For this review, take the finished solid that the model builds, in its own axes (mm). A direction names the side the tool comes from. Give positions to 0.01 mm unless a question says otherwise; leave off trailing zeros. Write each loop counter-clockwise with the first axis right and the second up, starting at its lowest first coordinate (ties: lowest second). Pieces come first, ordered by that corner, then holes.
Q1. We need section D-D (z = 0.1). Write out the cut boundary in (x, y).
Q2. We need section C-C (x = 1.1). Write out the cut boundary in (y, z).
Q3. We need section A-A (z = -3.55). Write out the cut boundary in (x, y) (3 decimals).
Q4. For line 1 (Y direction, x = -0.5, z = -4.15); line 2 (Y direction, x = -0.3, z = -2.25); line 3 (Z direction, x = 0, y = 1), list the stretches that pass through material, from the lowest coordinate up.
Q5. Machinability: for faces 5 (the flat face through (0.5, 7.3, -2.75)), 6 (the flat face through (0, 3, -0.75)), 7 (the flat face through (-0.5, 3, 0)), which of the approach directions +Z, -Z, +X, -X, +Y, -Y give a long, thin tool a straight path to every point of the face, cutting with its end or side? Answer none if there is none.
Q6. Mouldability with a two-part tool opening along Z and no side actions: class faces 1 (the cylindrical face through (-0.133, 1.479, -0.167)), 2 (the flat face through (0.5, 3, 0)), 3 (the flat face through (-1.25, 5, 0)), 4 (the cylindrical face through (-0.018, 6.199, -1.035)) as released by +Z, released by -Z, zero draft, split by the parting line, or undercut.
Q7. We need section B-B (y = 0.75). Write out the cut boundary in (x, z) (3 decimals).
Q8. Insertion check: P1, Ø0.8, axis at x = 0, z = -3, coming from the -Y side; P2, Ø1, axis at x = 0.5, z = 0, coming from the -Y side; P3, Ø2, axis at y = 4, z = -2.5, coming from the -X side; P4, Ø1, axis at x = -1, z = -1.5, coming from the -Y side. Each pin has a flat end and moves straight along its axis. Give the tip position at first contact, or say it passes through.
```python
from build123d import *

# Parameters (mm, degrees)
SKETCH_1_W          = 2.5
SKETCH_1_H          = 1.5
EXTRUDE_1_DEPTH     = 8
SKETCH_5_R          = 0.435
CUT_EXTRUDE_1_DEPTH = 3
SKETCH_6_W          = 2.5
SKETCH_6_H          = 1.5
EXTRUDE_2_DEPTH     = 4
FILLET_1_R          = 1
SKETCH_7_R          = 0.435
CUT_EXTRUDE_2_DEPTH = 2


with BuildPart() as part:
    # Эскиз1 → Бобышка-Вытянуть1 (new body)
    with BuildSketch(Plane(origin=(0, 0, 0), x_dir=(1, 0, 0), z_dir=(0, 1, 0))):
        Rectangle(SKETCH_1_W, SKETCH_1_H)
    extrude(amount=EXTRUDE_1_DEPTH)

    # Эскиз5 → Вырез-Вытянуть1 (cut)
    with BuildSketch(Plane.XZ):
        with Locations((0.535, 0)):
            Circle(SKETCH_5_R)
        with Locations((-0.535, 0)):
            Circle(SKETCH_5_R)
    extrude(amount=-CUT_EXTRUDE_1_DEPTH, mode=Mode.SUBTRACT)

    # Эскиз6 → Бобышка-Вытянуть2 (add)
    with BuildSketch(Plane(origin=(0, 0, -0.75), x_dir=(-1, 0, 0), z_dir=(0, 0, -1))):
        with Locations((0, 7.25)):
            Rectangle(SKETCH_6_W, SKETCH_6_H)
    extrude(amount=EXTRUDE_2_DEPTH)

    # Скругление1
    fillet_1_edges = [part.edges().sort_by_distance(p)[0] for p in [
        (0, 8, 0.75),
        (0, 6.5, -0.75),
    ]]
    fillet(fillet_1_edges, radius=FILLET_1_R)

    # Эскиз7 → Вырез-Вытянуть2 (cut)
    with BuildSketch(Plane(origin=(0, 0, -4.75), x_dir=(-1, 0, 0), z_dir=(0, 0, -1))):
        with Locations((-0.535, 7.25)):
            Circle(SKETCH_7_R)
        with Locations((0.535, 7.25)):
            Circle(SKETCH_7_R)
    extrude(amount=-CUT_EXTRUDE_2_DEPTH, mode=Mode.SUBTRACT)


solid = part.part
```
Computed:
1. outline: (-1.25, 0) - (-0.96, 0) - (-0.96, 3) - (-0.11, 3) - (-0.11, 0) - (0.11, 0) - (0.11, 3) - (0.96, 3) - (0.96, 0) - (1.25, 0) - (1.25, 7.94) - (-1.25, 7.94) - close
2. outline: (0, -0.75) - (5.5, -0.75) arc R1 cw to (6.5, -1.75) - (6.5, -4.75) - (8, -4.75) - (8, -0.25) arc R1 ccw to (7, 0.75) - (0, 0.75) - close
3. outline: (-1.25, 6.5) - (1.25, 6.5) - (1.25, 8) - (-1.25, 8) - close; hole circle Ø0.87 at (-0.535, 7.25); hole circle Ø0.87 at (0.535, 7.25)
4. line 1: y = 6.5 to 6.82, 7.68 to 8
4. line 2: y = 6.5 to 8
4. line 3: z = -0.75 to 0.75
5. face 5: -Z
5. face 6: -Z, +X, -X, -Y
5. face 7: -Y
6. face 1: undercut
6. face 2: undercut
6. face 3: zero draft
6. face 4: released by -Z
7. outline: (-1.25, -0.75) - (1.25, -0.75) - (1.25, 0.75) - (-1.25, 0.75) - close; hole circle Ø0.87 at (-0.535, 0); hole circle Ø0.87 at (0.535, 0)
8. P1: stops at y = 6.5
8. P2: stops at y = 0
8. P3: passes through
8. P4: stops at y = 6.16
